from build123d import *

# Parameters (mm, degrees)
SKETCH1_R            = 10
BOSS_EXTRUDE1_DEPTH  = 255
SKETCH2_R            = 5
CUT_EXTRUDE1_DEPTH   = 250
BOSS_EXTRUDE2_START  = -10
SKETCH3_R            = 10
BOSS_EXTRUDE2_DEPTH  = 50
BOSS_EXTRUDE3_DEPTH  = 10
BOSS_EXTRUDE4_START  = -40
BOSS_EXTRUDE4_DEPTH  = 10
BOSS_EXTRUDE6_START  = 10
SKETCH5_W            = 35
SKETCH5_H            = 30
BOSS_EXTRUDE6_DEPTH  = 10
SKETCH6_W            = 35
SKETCH6_H            = 30
BOSS_EXTRUDE8_DEPTH  = 11
SKETCH7_R            = 6
CUT_EXTRUDE2_DEPTH   = 21
SKETCH8_R            = 2.5
BOSS_EXTRUDE9_DEPTH  = 4
SKETCH9_R            = 10
SKETCH9_R_2          = 7.5
SKETCH9_R_3          = 2.5
CUT_EXTRUDE3_DEPTH   = 3
SKETCH10_R           = 2
BOSS_EXTRUDE10_DEPTH = 5


with BuildPart() as part:
    # Sketch1 → Boss-Extrude1 (new body)
    with BuildSketch(Plane.XY):
        Circle(SKETCH1_R)
    extrude(amount=BOSS_EXTRUDE1_DEPTH)

    # Sketch2 → Cut-Extrude1 (cut)
    with BuildSketch(Plane.XY.offset(255)):
        Circle(SKETCH2_R)
    extrude(amount=-CUT_EXTRUDE1_DEPTH, mode=Mode.SUBTRACT)

    # Sketch3 → Boss-Extrude2 (add)
    with BuildSketch(Plane(origin=(0, 0, 0), x_dir=(-1, 0, 0), z_dir=(0, 0, -1)).offset(BOSS_EXTRUDE2_START)):
        Polygon((17.320508076, 0), (8.660254038, 15), (-8.660254038, 15), (-17.320508076, 0), (-8.660254038, -15), (8.660254038, -15), align=None)
        Circle(SKETCH3_R, mode=Mode.SUBTRACT)
    extrude(amount=-BOSS_EXTRUDE2_DEPTH)

    # Sketch4 → Boss-Extrude3 (add)
    with BuildSketch(Plane(origin=(0, 0, 10), x_dir=(-1, 0, 0), z_dir=(0, 0, -1))):
        Polygon((-9.526279442, -16.5), (9.526279442, -16.5), (19.052558883, 0), (9.526279442, 16.5), (-9.526279442, 16.5), (-19.052558883, 0), align=None)
        Polygon((8.660254038, 15), (-8.660254038, 15), (-17.320508076, 0), (-8.660254038, -15), (8.660254038, -15), (17.320508076, 0), align=None, mode=Mode.SUBTRACT)
    extrude(amount=-BOSS_EXTRUDE3_DEPTH)

    # Sketch4_2 → Boss-Extrude4 (add)
    with BuildSketch(Plane(origin=(0, 0, 10), x_dir=(-1, 0, 0), z_dir=(0, 0, -1)).offset(BOSS_EXTRUDE4_START)):
        Polygon((-9.526279442, -16.5), (9.526279442, -16.5), (19.052558883, 0), (9.526279442, 16.5), (-9.526279442, 16.5), (-19.052558883, 0), align=None)
        Polygon((8.660254038, 15), (-8.660254038, 15), (-17.320508076, 0), (-8.660254038, -15), (8.660254038, -15), (17.320508076, 0), align=None, mode=Mode.SUBTRACT)
    extrude(amount=-BOSS_EXTRUDE4_DEPTH)



with BuildPart() as body_2:
    # Sketch5 → Boss-Extrude6 (new body)
    with BuildSketch(Plane(origin=(10, 0, 0), x_dir=(0, 0, -1), z_dir=(1, 0, 0)).offset(BOSS_EXTRUDE6_START)):
        with Locations((-77.5, 1.5)):
            Rectangle(SKETCH5_W, SKETCH5_H)
    extrude(amount=BOSS_EXTRUDE6_DEPTH)


with BuildPart() as part_1:
    add(part.part)

    add(body_2.part)  # Boss-Extrude8 merges body 2
    # Sketch6 → Boss-Extrude8 (add)
    with BuildSketch(Plane.ZY.offset(-20)):
        with Locations((77.5, 1.5)):
            Rectangle(SKETCH6_W, SKETCH6_H)
    extrude(amount=BOSS_EXTRUDE8_DEPTH)

    # Sketch7 → Cut-Extrude2 (cut)
    with BuildSketch(Plane(origin=(0, 16.5, 0), x_dir=(1, 0, 0), z_dir=(0, 1, 0))):
        with Locations((19.5, -85)):
            Circle(SKETCH7_R)
    extrude(amount=-CUT_EXTRUDE2_DEPTH, mode=Mode.SUBTRACT)

    # Sketch8 → Boss-Extrude9 (add)
    with BuildSketch(Plane.ZY.offset(-9)):
        with Locations((90, 11.5)):
            Circle(SKETCH8_R)
    extrude(amount=BOSS_EXTRUDE9_DEPTH)

    # Sketch9 → Cut-Extrude3 (cut)
    with BuildSketch(Plane(origin=(30, 0, 0), x_dir=(0, 0, -1), z_dir=(1, 0, 0))):
        with Locations((-83, 4.5)):
            Circle(SKETCH9_R)
        with Locations((-83, 4.5)):
            Circle(SKETCH9_R_2, mode=Mode.SUBTRACT)
        with Locations((-83, 4.5)):
            Circle(SKETCH9_R_3)
    extrude(amount=-CUT_EXTRUDE3_DEPTH, mode=Mode.SUBTRACT)

    # Sketch10 → Boss-Extrude10 (add)
    with BuildSketch(Plane(origin=(30, 0, 0), x_dir=(0, 0, -1), z_dir=(1, 0, 0))):
        with Locations((-92, 13.5)):
            Circle(SKETCH10_R)
    extrude(amount=BOSS_EXTRUDE10_DEPTH)


solid = part_1.part
Work out the finished part from the listing and answer in its coordinate system (mm). A direction names the side the tool comes from. Round coordinates to 2 decimals unless told otherwise and drop trailing zeros. Loops run counter-clockwise (first coordinate to the right, second up) from the corner with the lowest first, then second, coordinate; pieces in that order, holes last. Notation, with made-up numbers: (-25, 33) -> (7, 33) arc R22 ccw to (7, 72) -> close; hole circle Ø10 at (25, 50). An arc over 180 degrees is marked (long way). Use one line per item in the form item = value.
(1) Straight lines are drawn through the part: line 1 (Y direction, x = 28.1, z = 83); line 2 (Z direction, x = 19, y = 0); line 3 (Z direction, x = 19.5, y = 1.25). For each, find the intervals that lie inside material, in ascending order.
Answer list:
line_1 = -13.5 to -5.5, -3 to 2, 7 to 12, 14.5 to 16.5
line_2 = 10 to 20, 50 to 79.02, 90.98 to 95
line_3 = 60 to 79, 91 to 95
(2) A tool of negligible diameter and unlimited length cuts with its end or side. For faces 4 (the cylindrical face through (18.72, 6.15, 79.05)), 5 (the flat face through (14.36, -8.13, 54.93)), 6 (the flat face through (27, 11.2, 79.3)), 7 (the flat face through (-14, 6.2, 50)), from which of +Z, -Z, +X, -X, +Y, -Y can it reach the whole face along a straight path? Write none if from no direction.
Answer list:
face_4 = +Y
face_5 = -Z, +X, -Y
face_6 = +X
face_7 = none
(3) Flat-ended cylindrical pins translate along their axes: P1, Ø6, axis at x = -7, z = 221.5, coming from the -Y side; P2, Ø11, axis at x = 2.5, y = 1, coming from the +Z side; P3, Ø8, axis at x = 21, y = 8, coming from the +Z side; P4, Ø5, axis at x = 1.5, z = 34, coming from the +Y side. Find the tip coordinate at first contact, or state that the pin passes through.
Answer list:
P1 = -9.17
P2 = 255
P3 = 95
P4 = 15
(4) For a pull along X with two mould halves and no side action, classify faces 1 (the flat face through (20, -13.5, 77)), 2 (the flat face through (9, 11, 77)), 3 (the cylindrical face through (-2.17, -9.76, 4.93)) as released by +X, released by -X, zero draft, split by the parting line, or undercut.
Answer list:
face_1 = zero draft
face_2 = undercut
face_3 = split by the parting line
(5) Find section A-A on z = 137. Give the vertices of the cut face in (x, y), then the cut area to 3 significant figures.
Answer list:
outline = circle Ø20 at (0, 0); hole circle Ø10 at (0, 0)
area = 236 mm2
(6) Find section B-B on x = -14.5. Give the vertices of the cut face in (y, z), then the cut area to 3 significant figures.
Answer list:
outline = (-7.89, 10) -> (7.89, 10) -> (7.89, 20) -> (4.89, 20) -> (4.89, 50) -> (7.89, 50) -> (7.89, 60) -> (-7.89, 60) -> (-7.89, 50) -> (-4.89, 50) -> (-4.89, 20) -> (-7.89, 20) -> close
area = 609 mm2
